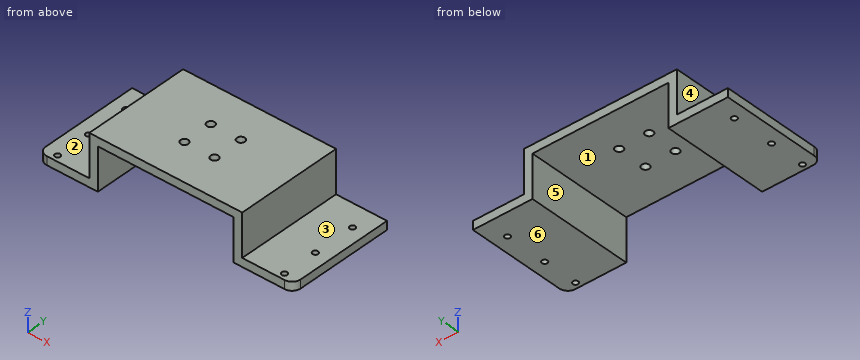
```python
from build123d import *

# Parameters (mm, degrees)
PAD008_DEPTH    = 63
FILLET003_R     = 5
SKETCH052_R     = 1.6
POCKET033_DEPTH = 5
SKETCH053_R     = 2.3
POCKET034_DEPTH = 5


with BuildPart() as part:
    # Sketch051 → Pad008 (new body)
    with BuildSketch(Plane.XZ):
        Polygon((-75, 0), (-75, 5), (-45, 5), (-45, 30), (45, 30), (45, 5), (75, 5), (75, 0), (40, 0), (40, 25), (-40, 25), (-40, 0), align=None)
    extrude(amount=PAD008_DEPTH)

    # Fillet003
    fillet003_edges = [part.edges().sort_by_distance(p)[0] for p in [
        (75, -63, 2.5),
        (-75, -63, 2.5),
    ]]
    fillet(fillet003_edges, radius=FILLET003_R)

    # Sketch052 (on Face11 of Fillet003) → Pocket033 (cut)
    with BuildSketch(Plane(origin=(0, 0, 5), x_dir=(-1, 0, 0), z_dir=(0, 0, 1))):
        with Locations((-66.75, 13.75)):
            Circle(SKETCH052_R)
        with Locations((-66.75, 38.75)):
            Circle(SKETCH052_R)
        with Locations((-66.75, 59.45)):
            Circle(SKETCH052_R)
        with Locations((66.75, 59.45)):
            Circle(SKETCH052_R)
        with Locations((66.75, 38.75)):
            Circle(SKETCH052_R)
        with Locations((66.75, 13.75)):
            Circle(SKETCH052_R)
    extrude(amount=-POCKET033_DEPTH, mode=Mode.SUBTRACT)

    # Sketch053 (on Face12 of Pocket033) → Pocket034 (cut)
    with BuildSketch(Plane(origin=(0, 0, 30), x_dir=(-1, 0, 0), z_dir=(0, 0, 1))):
        with Locations((8.8388347648, 40.3388347648)):
            Circle(SKETCH053_R)
        with Locations((8.8388347648, 22.6611652352)):
            Circle(SKETCH053_R)
        with Locations((-8.8388347648, 22.6611652352)):
            Circle(SKETCH053_R)
        with Locations((-8.8388347648, 40.3388347648)):
            Circle(SKETCH053_R)
    extrude(amount=-POCKET034_DEPTH, mode=Mode.SUBTRACT)


solid = part.part
```
Geometry: final body of the model. Coordinates: model frame, mm. Face numbers are marked on the shaded views. A direction names the side the tool comes from. Round coordinates to 2 decimals unless told otherwise and drop trailing zeros. Write each loop counter-clockwise with the first axis right and the second up, starting at its lowest first coordinate (ties: lowest second). Pieces come first, ordered by that corner, then holes.
Item 1: Mould query, pull axis X, two halves, no side actions, for the marked faces 4, 5 and 6. Classes: +X half, -X half, draft (parallel to the pull), parting line (faces both ways), or undercut.
Item 2: Section query C-C (z = 15.5). Return loops of the section in (x, y), plus the area to 3 significant figures.
Item 3: Pin query (flat end, axial travel): P1, Ø24, axis at x = -62, y = -24, coming from the +Z side; P2, Ø2, axis at x = -21, y = -28, coming from the -Z side; P3, Ø7.5, axis at y = -16, z = 12, coming from the -X side. Return the tip coordinate at first contact, or that it passes through.
Item 4: Section query B-B (x = -66.75). Return loops of the section in (y, z), plus the area to 3 significant figures.
Item 5: Section query D-D (y = -51.5). Return loops of the section in (x, z), plus the area to 3 significant figures.
Item 6: Material intervals for L1, parallel to Y at x = -66.75, z = 3.35; L2, parallel to X at y = -55, z = 9.25; L3, parallel to X at y = -38.75, z = 1.2, sorted ascending.
Item 7: Section query A-A (y = -13.75). Return loops of the section in (x, z).
Item 8: Set-up query: the marked faces 1, 2 and 3. Return all of +Z, -Z, +X, -X, +Y, -Y with unobstructed straight access to the full face (end or side cutting, diameter ignored); none if empty.
Completed:
1. face 4: -X half
1. face 5: undercut
1. face 6: draft
2. outline: (-45, -63) - (-40, -63) - (-40, 0) - (-45, 0) - close; (40, -63) - (45, -63) - (45, 0) - (40, 0) - close
2. area: 630 mm2
3. P1: stops at z = 5
3. P2: stops at z = 25
3. P3: stops at x = -45
4. outline: (-63, 0) - (-61.05, 0) - (-61.05, 5) - (-63, 5) - close; (-57.85, 0) - (-40.35, 0) - (-40.35, 5) - (-57.85, 5) - close; (-37.15, 0) - (-15.35, 0) - (-15.35, 5) - (-37.15, 5) - close; (-12.15, 0) - (0, 0) - (0, 5) - (-12.15, 5) - close
4. area: 267 mm2
5. outline: (-75, 0) - (-40, 0) - (-40, 25) - (40, 25) - (40, 0) - (75, 0) - (75, 5) - (45, 5) - (45, 30) - (-45, 30) - (-45, 5) - (-75, 5) - close
5. area: 1,000 mm2
6. L1: y = -63 to -61.05, -57.85 to -40.35, -37.15 to -15.35, -12.15 to 0
6. L2: x = -45 to -40, 40 to 45
6. L3: x = -75 to -68.35, -65.15 to -40, 40 to 65.15, 68.35 to 75
7. outline: (-75, 0) - (-68.35, 0) - (-68.35, 5) - (-75, 5) - close; (-65.15, 0) - (-40, 0) - (-40, 25) - (40, 25) - (40, 0) - (65.15, 0) - (65.15, 5) - (45, 5) - (45, 30) - (-45, 30) - (-45, 5) - (-65.15, 5) - close; (68.35, 0) - (75, 0) - (75, 5) - (68.35, 5) - close
8. face 1: -Z, +Y, -Y
8. face 2: +Z, -X, +Y, -Y
8. face 3: +Z, +X, +Y, -Y
